```python
from build123d import *

# Parameters (mm, degrees)
F1_DEPTH = 580
F2_R     = 5.5
F3_DEPTH = 40.001


with BuildPart() as f1:
    # F0 (on Front) → F1 (new body)
    with BuildSketch(Plane.XZ):
        Polygon((123.124914, 24.05611), (-124.875086, 24.05611), (-124.875086, -5.94389), (-69.875086, -5.94389), (-69.875086, -15.94389), (68.124914, -15.94389), (68.124914, -5.94389), (123.124914, -5.94389), align=None)
    extrude(amount=F1_DEPTH)

    # F2 (on face) → F3 (cut, through all)
    with BuildSketch(Plane.XY.offset(24.05611)):
        with Locations((-87.375086, -25)):
            Circle(F2_R)
        with Locations((85.624914, -25)):
            Circle(F2_R)
        with Locations((-87.375086, -157.5)):
            Circle(F2_R)
        with Locations((85.624914, -157.5)):
            Circle(F2_R)
        with Locations((-87.375086, -290)):
            Circle(F2_R)
        with Locations((85.624914, -290)):
            Circle(F2_R)
        with Locations((-87.375086, -422.5)):
            Circle(F2_R)
        with Locations((85.624914, -422.5)):
            Circle(F2_R)
        with Locations((85.624914, -555)):
            Circle(F2_R)
        with Locations((-87.375086, -555)):
            Circle(F2_R)
    extrude(amount=-F3_DEPTH, mode=Mode.SUBTRACT)


solid = f1.part
```
Geometry: final body of the model. Coordinates: model frame, mm. A direction names the side the tool comes from. Round coordinates to 2 decimals unless told otherwise and drop trailing zeros. Write each loop counter-clockwise with the first axis right and the second up, starting at its lowest first coordinate (ties: lowest second). Pieces come first, ordered by that corner, then holes. Notation, with made-up numbers: (81.25, 15) -> (101.25, 15) arc R27 ccw to (101.25, 48) -> close; hole circle Ø8 at (52, 63.5). An arc over 180 degrees is marked (long way). Return JSON: item names as keys, results as strings.
Q1. First-contact query: pin 1 Ø10 at (x, y) = (85.62, -290) entering from +Z; pin 2 Ø5 at (y, z) = (-355.5, -13.5) entering from +X; pin 3 Ø3 at (y, z) = (-263, -13) entering from -X; pin 4 Ø17.5 at (x, y) = (-87.38, -157.5) entering from -Z. Flat tips, straight axial feed; report the tip coordinate or a pass-through.
From the geometry:
{"pin 1": "through", "pin 2": "x = 68.12", "pin 3": "x = -69.88", "pin 4": "z = -5.94"}
Q2. Ray query, line 1 (X direction, y = -422, z = 10); line 2 (Y direction, x = 81.5, z = -2.5); line 3 (X direction, y = -426.5, z = 20.5). Return the intervals inside material, ascending.
From the geometry:
{"line 1": "-124.88 to -92.85, -81.9 to 80.15, 91.1 to 123.12", "line 2": "-580 to -558.64, -551.36 to -426.14, -418.86 to -293.64, -286.36 to -161.14, -153.86 to -28.64, -21.36 to 0", "line 3": "-124.88 to -91.15, -83.6 to 81.85, 89.4 to 123.12"}
Q3. Set-up query: faces 4 (the flat face through (1, -286, 24.056)), 5 (the flat face through (-69.875, -286, -11)), 6 (the flat face through (95, -286, -5.944)). Return all of +Z, -Z, +X, -X, +Y, -Y with unobstructed straight access to the full face (end or side cutting, diameter ignored); none if empty.
From the geometry:
{"face 4": "+Z, +X, -X, +Y, -Y", "face 5": "-Z, -X, +Y, -Y", "face 6": "-Z, +X, +Y, -Y"}
Q4. Section C-C on x = -108. Return the cut outline in (y, z).
From the geometry:
{"outline": "(-580, -5.94) -> (0, -5.94) -> (0, 24.06) -> (-580, 24.06) -> close"}
Q5. Section B-B on y = -306. Return the cut outline in (x, z).
From the geometry:
{"outline": "(-124.88, -5.94) -> (-69.88, -5.94) -> (-69.88, -15.94) -> (68.12, -15.94) -> (68.12, -5.94) -> (123.12, -5.94) -> (123.12, 24.06) -> (-124.88, 24.06) -> close"}
Q6. Mould query, pull axis X, two halves, no side actions, for faces 1 (the cylindrical face through (-92.87, -24.76, 9.27)), 2 (the flat face through (-3, -580, 4)), 3 (the flat face through (-124.875, -286, 9)). Classes: +X half, -X half, draft (parallel to the pull), parting line (faces both ways), or undercut.
From the geometry:
{"face 1": "undercut", "face 2": "draft", "face 3": "-X half"}
Q7. Section A-A on y = -555. Return the cut outline in (x, z), and give its area (3 significant figures).
From the geometry:
{"outline": "(-124.88, -5.94) -> (-92.88, -5.94) -> (-92.88, 24.06) -> (-124.88, 24.06) -> close; (-81.88, -5.94) -> (-69.88, -5.94) -> (-69.88, -15.94) -> (68.12, -15.94) -> (68.12, -5.94) -> (80.12, -5.94) -> (80.12, 24.06) -> (-81.88, 24.06) -> close; (91.12, -5.94) -> (123.12, -5.94) -> (123.12, 24.06) -> (91.12, 24.06) -> close", "area": "8,160 mm2"}
